from build123d import *

# Parameters (mm, degrees)
CUT_EXTRUDE4_DEPTH           = 66.955911542
CUT_EXTRUDE4_DEPTH_BACK      = 66.955911542
SKETCH3_R                    = 3.175
FILLET3_R                    = 6.35
BOSS_EXTRUDE1_START          = 9.8044
BOSS_EXTRUDE1_DEPTH          = 10.16
FILLET2_R                    = 3.175
CHAMFER2_SIZE                = 2.38125
CHAMFER2_SIZE_2              = 1.374815329
CUT_EXTRUDE3_DEPTH           = 63.420823637
CUT_EXTRUDE3_DEPTH_BACK      = 63.420823637
SKETCH8_R                    = 0.79375
F_5_16_24_TAPPED_HOLE1_D     = 6.9088
F_5_16_24_TAPPED_HOLE1_DEPTH = 12.7
F_5_16_24_TAPPED_HOLE1_TIP   = 2.075612922
CHAMFER3_SIZE                = 2.032
CHAMFER3_SIZE2               = 1.173175747


with BuildPart() as part:
    # Sketch1 → Revolve1 (revolve)
    with BuildSketch(Plane.XY, mode=Mode.PRIVATE) as revolve1_sk:
        Polygon((10.31875, 19.9644), (14.2875, 19.9644), (14.2875, 9.8044), (44.45, 9.8044), (44.45, 5.0419), (28.575, 5.0419), (25.1206, 1.5875), (25.1206, 0), (10.31875, 0), align=None)
    revolve(revolve1_sk.sketch.rotate(Axis((0, 0, 0), (0, 1, 0)), 90), axis=Axis((0, 0, 0), (0, 1, 0)))

    # Sketch3 → Cut-Extrude4 (cut, two sides: drawn at the far end of the back side and taken through both)
    with BuildSketch(Plane(origin=(0, 0, 0), x_dir=(1, 0, 0), z_dir=(0, 1, 0)).offset(-CUT_EXTRUDE4_DEPTH_BACK)):
        with BuildLine():
            Line((0, -44.45), (-44.45, 0))
            ThreePointArc((-44.45, 0), (-31.430896424, -31.430896424), (0, -44.45))
        make_face()
        with BuildLine():
            Line((44.45, 0), (0, -44.45))
            ThreePointArc((0, -44.45), (31.430896424, -31.430896424), (44.45, 0))
        make_face()
        with BuildLine():
            ThreePointArc((44.45, 0), (31.430896424, 31.430896424), (0, 44.45))
            Line((0, 44.45), (44.45, 0))
        make_face()
        with BuildLine():
            ThreePointArc((0, 44.45), (-31.430896424, 31.430896424), (-44.45, 0))
            Line((-44.45, 0), (0, 44.45))
        make_face()
        with Locations(Location((-34.29, 0, 0), (0, 0, 270))):
            Circle(SKETCH3_R)
        with Locations(Location((0, 34.29, 0), (0, 0, 270))):
            Circle(SKETCH3_R)
        with Locations(Location((34.29, 0, 0), (0, 0, 270))):
            Circle(SKETCH3_R)
        with Locations(Location((0, -34.29, 0), (0, 0, 270))):
            Circle(SKETCH3_R)
    extrude(amount=CUT_EXTRUDE4_DEPTH + CUT_EXTRUDE4_DEPTH_BACK, mode=Mode.SUBTRACT)

    # Fillet3
    fillet3_edges = [part.edges().sort_by_distance(p)[0] for p in [
        (0, 7.42315, -44.45),
        (44.45, 7.42315, 0),
        (0, 7.42315, 44.45),
        (-44.45, 7.42315, 0),
    ]]
    fillet(fillet3_edges, radius=FILLET3_R)

    # Sketch4 → Boss-Extrude1 (add)
    with BuildSketch(Plane(origin=(0, 0, 0), x_dir=(1, 0, 0), z_dir=(0, 1, 0)).offset(BOSS_EXTRUDE1_START)):
        Polygon((-22.225, 22.225), (-26.715128061, 17.734871939), (-11.786586159, 2.806330038), (-2.806330038, 11.786586159), (-17.734871939, 26.715128061), align=None)
    extrude(amount=BOSS_EXTRUDE1_DEPTH)

    # Fillet2
    fillet2_edges = [part.edges().sort_by_distance(p)[0] for p in [
        (10.102788136, 9.8044, 10.102788136),
        (-11.147443158, 9.8044, -20.127699279),
        (-20.127699279, 9.8044, -11.147443158),
    ]]
    fillet(fillet2_edges, radius=FILLET2_R)

    # Chamfer2
    # the kernel refuses this chamfer: 2.38125, 1.374815329 mm, written as the material it takes off along each edge
    with BuildSketch(Plane(origin=(0, 19.9644, 0), x_dir=(0, 0, -1), z_dir=(1, 0, 0))) as chamfer2_piece_1:
        Polygon((10.31875 + CHAMFER2_SIZE, 0), (10.31875, -CHAMFER2_SIZE_2), (10.31875, 0), align=None)
    revolve(axis=Axis((0, 19.9644, 0), (0, 1, 0)), revolution_arc=45.000000179, mode=Mode.SUBTRACT)
    with BuildSketch(Plane(origin=(0, 19.9644, 0), x_dir=(-0.7071067833935745, 0, -0.7071067789795206), z_dir=(0.7071067789795206, 0, -0.7071067833935745))) as chamfer2_piece_2:
        Polygon((10.31875 + CHAMFER2_SIZE, 0), (10.31875, -CHAMFER2_SIZE_2), (10.31875, 0), align=None)
    revolve(axis=Axis((0, 19.9644, 0), (0, 1, 0)), revolution_arc=314.999999821, mode=Mode.SUBTRACT)

    # Sketch8 → Cut-Extrude3 (cut, two sides: drawn at the far end of the back side and taken through both)
    with BuildSketch(Plane(origin=(0, 0, 0), x_dir=(1, 0, 0), z_dir=(0, 1, 0)).offset(-CUT_EXTRUDE3_DEPTH_BACK)):
        with Locations(Location((-17.06248663, 17.06248663, 0), (0, 0, 270))):
            Circle(SKETCH8_R)
    extrude(amount=CUT_EXTRUDE3_DEPTH + CUT_EXTRUDE3_DEPTH_BACK, mode=Mode.SUBTRACT)

    # 5/16-24 Tapped Hole1
    with Locations(Plane(origin=(0, 19.9644, 0), x_dir=(1, 0, 0), z_dir=(0, 1, 0))):
        with Locations((-18.183884746, 18.183884746)):
            Hole(F_5_16_24_TAPPED_HOLE1_D / 2, depth=F_5_16_24_TAPPED_HOLE1_DEPTH)
            with Locations((0, 0, -(F_5_16_24_TAPPED_HOLE1_DEPTH + F_5_16_24_TAPPED_HOLE1_TIP / 2))):  # 118° drill point
                Cone(0, F_5_16_24_TAPPED_HOLE1_D / 2, F_5_16_24_TAPPED_HOLE1_TIP, mode=Mode.SUBTRACT)

    # Chamfer3
    chamfer3_edges = [part.edges().sort_by_distance(p)[0] for p in [
        (-14.729484746, 19.9644, -18.183884746),
    ]]
    chamfer3_side = [part.faces().sort_by_distance(p)[0] for p in [
        (-9.027932252, 19.9644, -9.027932252),
    ]]
    chamfer(chamfer3_edges, length=CHAMFER3_SIZE, length2=CHAMFER3_SIZE2, reference=chamfer3_side[0])


solid = part.part
Can you work these out from the model? Positions are in its coordinate system, mm. A direction names the side the tool comes from. Round coordinates to 2 decimals unless told otherwise and drop trailing zeros. Write each loop counter-clockwise with the first axis right and the second up, starting at its lowest first coordinate (ties: lowest second). Pieces come first, ordered by that corner, then holes. Notation, with made-up numbers: (-13, 37.5) - (1, 37.5) arc R20 ccw to (1, 76.5) - close; hole circle Ø7 at (-20, 15). An arc over 180 degrees is marked (long way). Write each question's results on one line, items separated by ' | '. Start each with the question number.
1) Suppose I cut it at A-A (z = -34.29). List the corners of the cut face in (x, y) for me (3 decimals), and give its area (3 significant figures).
2) Please list where these lines run through material, in increasing order: line 1 (X direction, y = 8.25, z = 0) (3 decimals); line 2 (X direction, y = 2.25, z = -2); line 3 (Y direction, x = 33.5, z = 7.5).
3) Suppose I cut it at C-C (z = 0). Give the number of separate pieces and of enclosed holes in the cut face, and give its area (3 significant figures).
4) Which directions (+Z, -Z, +X, -X, +Y, -Y) give clear straight access to the entire face, cutting with the end or side of a thin tool? Please do faces 1 (the cylindrical face through (-10.23, 9.42, 1.34)), 2 (the flat face through (-19, 5.042, 22)).
5) We'd pull the mould along Z, two halves only. Please class faces 3 (the cylindrical face through (-0.07, 7.46, 41.82)), 4 (the cylindrical face through (-10.6, 10.76, -20.86)), 5 (the cylindrical face through (0.95, 7.39, -31.26)), 6 (the flat face through (11, 0, 0)): released by +Z, released by -Z, zero draft, split by the parting line, or undercut.
6) For pin 1 Ø10 at (y, z) = (9.5, 31.5) entering from -X; pin 2 Ø5 at (x, z) = (34.29, 0) entering from -Y; pin 3 Ø1 at (x, z) = (-4, -30.5) entering from +Y; pin 4 Ø8 at (x, z) = (-18.18, -18.18) entering from +Y, each with a flat end and sliding along its axis, tell me the tip position at first contact or that it passes through.
7) Suppose I cut it at B-B (x = -34.29). List the corners of the cut face in (y, z) for me (3 decimals).
Here are the results:
1) outline: (-10.16, 5.042) - (-3.175, 5.042) - (-3.175, 9.804) - (-10.16, 9.804) - close; (3.175, 5.042) - (10.16, 5.042) - (10.16, 9.804) - (3.175, 9.804) - close | area: 66.5 mm2
2) line 1: x = -41.82 to -37.465, -31.115 to -10.319, 10.319 to 31.115, 37.465 to 41.82 | line 2: x = -25.71 to -10.12, 10.12 to 25.71 | line 3: y = 5.04 to 9.8
3) separate pieces: 4 | enclosed holes: 0 | area: 482 mm2
4) face 1: +Y, -Y | face 2: -Y
5) face 3: released by +Z | face 4: released by -Z | face 5: undercut | face 6: zero draft
6) pin 1: stops at x = -17.95 | pin 2: passes through | pin 3: stops at y = 9.8 | pin 4: stops at y = 19.11
7) outline: (5.042, -10.16) - (9.804, -10.16) - (9.804, -3.175) - (5.042, -3.175) - close; (5.042, 3.175) - (9.804, 3.175) - (9.804, 10.16) - (5.042, 10.16) - close
